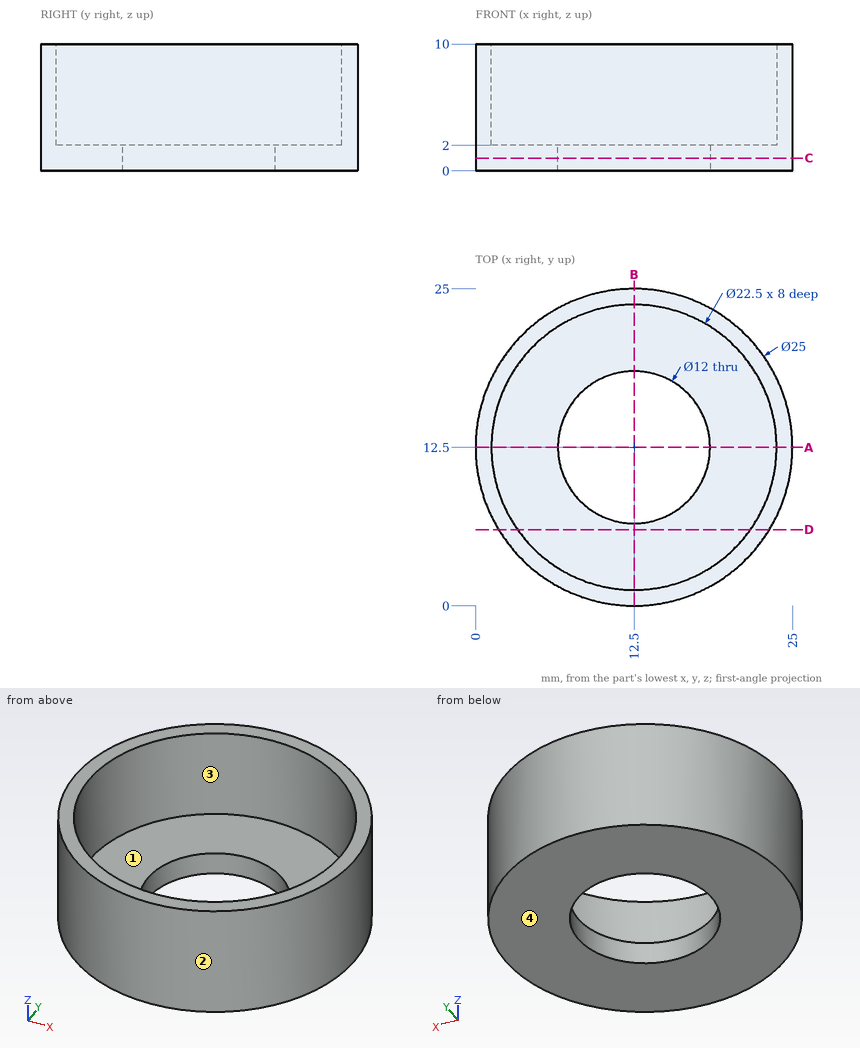
The figure shows three views and two pictorial views of one solid part (mm, origin at its lowest corner). Answer the questions. Coordinates: 2 decimals unless noted, no trailing zeros. Loops run counter-clockwise (first coordinate to the right, second up) from the corner with the lowest first, then second, coordinate; pieces in that order, holes last.
1) Find section C-C on z = 1. Write down the section's boundary in (x, y), then the cut area to 3 significant figures.
2) Determine the mould class of the marked faces 1, 2, 3 and 4 for opening direction Y: pulls with the +Y half, pulls with the -Y half, needs draft (parallel to the pull), parting line crosses it, or undercut.
3) Flat-ended cylindrical pins translate along their axes: pin 1 Ø1 at (y, z) = (17.5, 2.5) entering from +X; pin 2 Ø4 at (x, z) = (19, 4.5) entering from +Y; pin 3 Ø2 at (x, z) = (22, 2.5) entering from -Y. Find the tip coordinate at first contact, or state that the pin passes through.
4) Find section A-A on y = 12.5. Write down the section's boundary in (x, z), then the cut area to 3 significant figures.
5) Find section D-D on y = 6. Write down the section's boundary in (x, z), then the cut area to 3 significant figures.
6) Find the intervals of material crossed by L1, parallel to Y at x = 12.5, z = 5.75; L2, parallel to Y at x = 12.5, z = 1.55; L3, parallel to Z at x = 20.5, y = 10.5, in increasing order.
Values:
1. outline: circle Ø25 at (12.5, 12.5); hole circle Ø12 at (12.5, 12.5)
1. area: 378 mm2
2. face 1: undercut
2. face 2: parting line crosses it
2. face 3: undercut
2. face 4: needs draft
3. pin 1: stops at x = 24.16
3. pin 2: stops at y = 24.16
3. pin 3: stops at y = 3.33
4. outline: (0, 0) - (6.5, 0) - (6.5, 2) - (1.25, 2) - (1.25, 10) - (0, 10) - close; (18.5, 0) - (25, 0) - (25, 10) - (23.75, 10) - (23.75, 2) - (18.5, 2) - close
4. area: 46.0 mm2
5. outline: (1.82, 0) - (23.18, 0) - (23.18, 10) - (21.68, 10) - (21.68, 2) - (3.32, 2) - (3.32, 10) - (1.82, 10) - close
5. area: 66.6 mm2
6. L1: y = 0 to 1.25, 23.75 to 25
6. L2: y = 0 to 6.5, 18.5 to 25
6. L3: z = 0 to 2
